Could you check a few things on this model? Use its own coordinates, in mm. Face numbers are marked on the shaded views. A direction names the side the tool comes from. Round coordinates to 2 decimals unless told otherwise and drop trailing zeros. Loops run counter-clockwise (first coordinate to the right, second up) from the corner with the lowest first, then second, coordinate; pieces in that order, holes last. Notation, with made-up numbers: M 49.5,-10 L 75.5,-10 A26 ccw 75.5,4 Z; hole C 81,56.5 d2. An arc over 180 degrees is marked long. One line per item, written item: value. Start each with the question number.
Q1. Imagine slicing it at A-A (x = 39.8). Please give me the cut outline in (y, z), then the cut area to 3 significant figures.
Q2. I'm going to push flat-ended pins straight in: pin 1 Ø2.5 at (y, z) = (-53, 27.5) entering from +X; pin 2 Ø6 at (x, y) = (-19.5, -38.5) entering from +Z; pin 3 Ø12.5 at (x, y) = (39.8, -49.8) entering from +Z; pin 4 Ø1.5 at (x, z) = (-26.5, 27.5) entering from -Y. Where does each tip first touch, or does it pass through?
Q3. Thinking about a two-plate mould opening in Y: for the marked faces 3, 4 and 5, which applies, released by +Y, released by -Y, zero draft, split by the parting line, or undercut?
Q4. Please list where these lines run through material, in increasing order: line 1 along Y through (x, z) = (39.8, 3.8); line 2 along X through (y, z) = (14, 8.75).
Q5. Imagine slicing it at D-D (x = -53.5). Please give me the cut outline in (y, z).
Q6. Imagine slicing it at B-B (y = -49.8). Please give me the cut outline in (x, z), then the cut area to 3 significant figures.
Q7. Imagine slicing it at C-C (z = 22.25). Please give me the cut outline in (x, y), then the cut area to 3 significant figures.
Q8. Which directions (+Z, -Z, +X, -X, +Y, -Y) give clear straight access to the entire face, cutting with the end or side of a thin tool? Please do the marked faces 1 and 2.
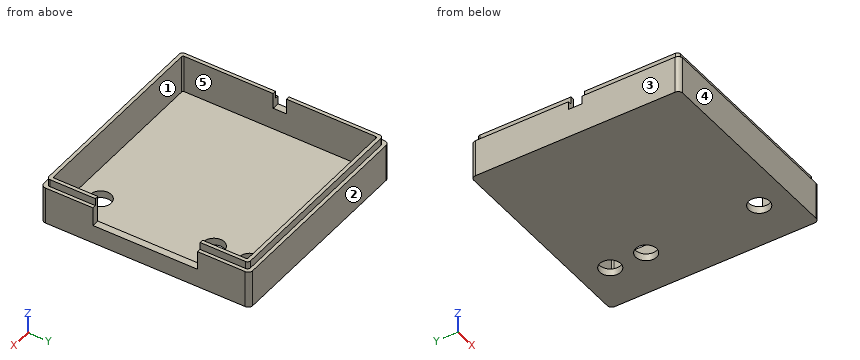
from build123d import *

# Parameters (mm, degrees)
SKETCH001_W     = 139.6
SKETCH001_H     = 139.6
PAD_DEPTH       = 25
SKETCH003_W     = 134.8
SKETCH003_H     = 134.8
PAD001_DEPTH    = 5
SKETCH002_W     = 130
SKETCH002_H     = 130
POCKET_DEPTH    = 25.2
SKETCH005_W     = 70
SKETCH005_H     = 17.6
POCKET001_DEPTH = 5
SKETCH006_W     = 9
SKETCH006_H     = 10.5
POCKET002_DEPTH = 5
SKETCH007_R     = 7
HOLE_DEPTH      = 25
FILLET_R        = 3
FILLET001_R     = 3
FILLET002_R     = 3
FILLET003_R     = 3
FILLET004_R     = 2
FILLET005_R     = 2
FILLET006_R     = 2
FILLET007_R     = 2
FILLET008_R     = 1
FILLET009_R     = 1
FILLET010_R     = 1
FILLET011_R     = 1


with BuildPart() as part:
    # Sketch001 → Pad (new body)
    with BuildSketch(Plane.XY):
        Rectangle(SKETCH001_W, SKETCH001_H)
    extrude(amount=PAD_DEPTH)

    # Sketch003 (on Face6 of Pad) → Pad001 (join)
    with BuildSketch(Plane.XY.offset(25)):
        Rectangle(SKETCH003_W, SKETCH003_H)
    extrude(amount=PAD001_DEPTH)

    # Sketch002 (on Face11 of Pad001) → Pocket (cut)
    with BuildSketch(Plane.XY.offset(30)):
        Rectangle(SKETCH002_W, SKETCH002_H)
    extrude(amount=-POCKET_DEPTH, mode=Mode.SUBTRACT)

    # Sketch005 (on Face3 of Pocket) → Pocket001 (cut)
    with BuildSketch(Plane.YZ.offset(69.8)):
        with Locations((0, 21.2)):
            Rectangle(SKETCH005_W, SKETCH005_H)
    extrude(amount=-POCKET001_DEPTH, mode=Mode.SUBTRACT)

    # Sketch006 (on Face2 of Pocket001) → Pocket002 (cut)
    with BuildSketch(Plane(origin=(-69.8, 0, 0), x_dir=(0, -1, 0), z_dir=(-1, 0, 0))):
        with Locations((0, 24.75)):
            Rectangle(SKETCH006_W, SKETCH006_H)
    extrude(amount=-POCKET002_DEPTH, mode=Mode.SUBTRACT)

    # Sketch007 (on Face25 of Pocket002) → Hole (cut)
    with BuildSketch(Plane.XY.offset(4.8)):
        with Locations((39.8, 49.8)):
            Circle(SKETCH007_R)
        with Locations((39.8, 25.8)):
            Circle(SKETCH007_R)
        with Locations((39.8, -49.8)):
            Circle(SKETCH007_R)
    extrude(amount=-HOLE_DEPTH, mode=Mode.SUBTRACT)

    # Fillet
    fillet_edges = [part.edges().sort_by_distance(p)[0] for p in [
        (-69.8, 69.8, 12.5),
    ]]
    fillet(fillet_edges, radius=FILLET_R)

    # Fillet001
    fillet001_edges = [part.edges().sort_by_distance(p)[0] for p in [
        (69.8, 69.8, 12.5),
    ]]
    fillet(fillet001_edges, radius=FILLET001_R)

    # Fillet002
    fillet002_edges = [part.edges().sort_by_distance(p)[0] for p in [
        (69.8, -69.8, 12.5),
    ]]
    fillet(fillet002_edges, radius=FILLET002_R)

    # Fillet003
    fillet003_edges = [part.edges().sort_by_distance(p)[0] for p in [
        (-69.8, -69.8, 12.5),
    ]]
    fillet(fillet003_edges, radius=FILLET003_R)

    # Fillet004
    fillet004_edges = [part.edges().sort_by_distance(p)[0] for p in [
        (-67.4, -67.4, 27.5),
    ]]
    fillet(fillet004_edges, radius=FILLET004_R)

    # Fillet005
    fillet005_edges = [part.edges().sort_by_distance(p)[0] for p in [
        (-67.4, 67.4, 27.5),
    ]]
    fillet(fillet005_edges, radius=FILLET005_R)

    # Fillet006
    fillet006_edges = [part.edges().sort_by_distance(p)[0] for p in [
        (67.4, 67.4, 27.5),
    ]]
    fillet(fillet006_edges, radius=FILLET006_R)

    # Fillet007
    fillet007_edges = [part.edges().sort_by_distance(p)[0] for p in [
        (67.4, -67.4, 27.5),
    ]]
    fillet(fillet007_edges, radius=FILLET007_R)

    # Fillet008
    fillet008_edges = [part.edges().sort_by_distance(p)[0] for p in [
        (-65, 65, 17.4),
    ]]
    fillet(fillet008_edges, radius=FILLET008_R)

    # Fillet009
    fillet009_edges = [part.edges().sort_by_distance(p)[0] for p in [
        (-65, -65, 17.4),
    ]]
    fillet(fillet009_edges, radius=FILLET009_R)

    # Fillet010
    fillet010_edges = [part.edges().sort_by_distance(p)[0] for p in [
        (65, -65, 17.4),
    ]]
    fillet(fillet010_edges, radius=FILLET010_R)

    # Fillet011
    fillet011_edges = [part.edges().sort_by_distance(p)[0] for p in [
        (65, 65, 17.4),
    ]]
    fillet(fillet011_edges, radius=FILLET011_R)


solid = part.part
Report:
1. outline: M -69.8,0 L -56.8,0 L -56.8,4.8 L -65,4.8 L -65,30 L -67.4,30 L -67.4,25 L -69.8,25 Z; M -42.8,0 L 18.8,0 L 18.8,4.8 L -42.8,4.8 Z; M 32.8,0 L 42.8,0 L 42.8,4.8 L 32.8,4.8 Z; M 56.8,0 L 69.8,0 L 69.8,25 L 67.4,25 L 67.4,30 L 65,30 L 65,4.8 L 56.8,4.8 Z
1. area: 686 mm²
2. pin 1: stops at x = 67.4
2. pin 2: stops at z = 4.8
2. pin 3: passes through
2. pin 4: stops at y = -67.4
3. face 3: zero draft
3. face 4: released by -Y
3. face 5: undercut
4. line 1: y = -69.8 to -56.8, -42.8 to 18.8, 32.8 to 42.8, 56.8 to 69.8
4. line 2: x = -69.8 to -65, 65 to 69.8
5. outline: M -69.8,0 L 69.8,0 L 69.8,25 L 67.4,25 L 67.4,30 L 65,30 L 65,4.8 L -65,4.8 L -65,30 L -67.4,30 L -67.4,25 L -69.8,25 Z
6. outline: M -69.8,0 L 32.8,0 L 32.8,4.8 L -65,4.8 L -65,30 L -67.4,30 L -67.4,25 L -69.8,25 Z; M 46.8,0 L 69.8,0 L 69.8,25 L 67.4,25 L 67.4,30 L 65,30 L 65,4.8 L 46.8,4.8 Z
6. area: 821 mm²
7. outline: M -69.8,-66.8 A3 ccw -66.8,-69.8 L 66.8,-69.8 A3 ccw 69.8,-66.8 L 69.8,-35 L 65,-35 L 65,-64 A1 cw 64,-65 L -64,-65 A1 cw -65,-64 L -65,-4.5 L -69.8,-4.5 Z; M -69.8,4.5 L -65,4.5 L -65,64 A1 cw -64,65 L 64,65 A1 cw 65,64 L 65,35 L 69.8,35 L 69.8,66.8 A3 ccw 66.8,69.8 L -66.8,69.8 A3 ccw -69.8,66.8 Z
7. area: 2,200 mm²
8. face 1: +Z
8. face 2: +Z, -Z, +X, -X, +Y
